```python
from build123d import *

# Parameters (mm, degrees)
F1_DEPTH = 40
F2_R     = 2


with BuildPart() as f1:
    # F0 (on Top) → F1 (new body)
    with BuildSketch(Plane.XY):
        Polygon((-3.5, 2.020726), (-3.5, -2.020726), (0, -4.041452), (3.5, -2.020726), (3.5, 2.020726), (0, 4.041452), align=None)
    extrude(amount=F1_DEPTH)

    # F2
    f2_edges = [f1.edges().sort_by_distance(p)[0] for p in [
        (-3.5, 0, 40),
        (-1.75, -3.031089, 40),
        (1.75, -3.031089, 40),
        (3.5, 0, 40),
        (1.75, 3.031089, 40),
        (-1.75, 3.031089, 40),
    ]]
    fillet(f2_edges, radius=F2_R)

    # F3 (on Right) → F4 (revolve, cut)
    with BuildSketch(Plane.YZ):
        Polygon((11.752745, 17.418522), (0, 0), (0, -5.376646), (19.7981, -5.376646), (22.114186, 17.418522), align=None)
    revolve(axis=Axis((0, 0, -2.688323), (0, 0, 1)), mode=Mode.SUBTRACT)


solid = f1.part
```
Geometry: final body of the model. Coordinates: model frame, mm. Coordinates: 2 decimals unless noted, no trailing zeros. Order: outer loops, then holes, each group sorted by start corner. A loop starts at its lowest first (then second) coordinate and runs counter-clockwise, first axis right, second up. Notation, with made-up numbers: (43.25, 40.25) - (88.25, 40.25) arc R24 cw to (88.25, 70.25) - close; hole circle Ø2 at (-33, -26.5). An arc over 180 degrees is marked (long way). Write each question's results on one line, items separated by ' | '.
1) Section A-A, the plane z = 15. Return loops of the section in (x, y), plus the area to 3 significant figures.
Results list:
outline: (-3.5, -2.02) - (0, -4.04) - (3.5, -2.02) - (3.5, 2.02) - (0, 4.04) - (-3.5, 2.02) - close | area: 42.4 mm^2
2) Line query: line 1 (Y direction, x = 2.75, z = 22.5); line 2 (X direction, y = -3, z = 14.5); line 3 (Z direction, x = 2.5, y = 1.75). Output: solid intervals per line, ascending. Write a range as from..to.
Results list:
line 1: -2.45..2.45 | line 2: -1.8..1.8 | line 3: 4.52..39.55
3) Pin query (flat end, axial travel): pin 1 (2 mm diameter, centred on x = -2, y = -3, fed in from -Z). Return the tip coordinate at first contact, or that it passes through.
Results list:
pin 1: z = 3.86
